Read the model definition and answer for the solid it produces. Units are mm, in the model's axes. A direction names the side the tool comes from. Coordinates: 2 decimals unless noted, no trailing zeros. Write each loop counter-clockwise with the first axis right and the second up, starting at its lowest first coordinate (ties: lowest second). Pieces come first, ordered by that corner, then holes. Notation, with made-up numbers: (62, 43.25) - (72, 43.25) arc R20 ccw to (72, 69.25) - close; hole circle Ø3 at (24, 59.25). An arc over 180 degrees is marked (long way). Return JSON: item names as keys, results as strings.
```python
from build123d import *

# Parameters (mm, degrees)
SKETCH_1_W      = 101
SKETCH_1_H      = 20
SKETCH_1_R      = 4
EXTRUDE_1_DEPTH = 3
EXTRUDE_2_DEPTH = 3
SKETCH_3_W      = 20
SKETCH_3_H      = 20
SKETCH_3_R      = 2
EXTRUDE_3_DEPTH = 3
SKETCH_4_W      = 95
SKETCH_4_H      = 20
EXTRUDE_4_DEPTH = 3
SKETCH_5_W      = 95
SKETCH_5_H      = 20
EXTRUDE_5_DEPTH = 3


with BuildPart() as part:
    # 草图1 → 凸台-拉伸1 (new body)
    with BuildSketch(Plane(origin=(0, 0, 0), x_dir=(1, 0, 0), z_dir=(0, 1, 0))):
        Rectangle(SKETCH_1_W, SKETCH_1_H)
        with Locations((-37.5, 0)):
            Circle(SKETCH_1_R, mode=Mode.SUBTRACT)
        with Locations((37.5, 0)):
            Circle(SKETCH_1_R, mode=Mode.SUBTRACT)
    extrude(amount=EXTRUDE_1_DEPTH)

    # 草图2 → 凸台-拉伸2 (add)
    with BuildSketch(Plane.ZY.offset(50.5)):
        Polygon((-10, 23), (-10, 3), (10, 3), (10, 23), (0, 23), align=None)
        with BuildLine():
            ThreePointArc((2, 13), (-1.414213562, 11.585786438), (0, 15))
            ThreePointArc((0, 15), (1.414213562, 14.414213562), (2, 13))
        make_face(mode=Mode.SUBTRACT)
    extrude(amount=-EXTRUDE_2_DEPTH)

    # 草图3 → 凸台-拉伸3 (add)
    with BuildSketch(Plane(origin=(50.5, 0, 0), x_dir=(0, 0, -1), z_dir=(1, 0, 0))):
        with Locations((0, 13)):
            Rectangle(SKETCH_3_W, SKETCH_3_H)
        with Locations((0, 13)):
            Circle(SKETCH_3_R, mode=Mode.SUBTRACT)
    extrude(amount=-EXTRUDE_3_DEPTH)

    # 草图4 → 凸台-拉伸4 (add)
    with BuildSketch(Plane.XY.offset(10)):
        with Locations((0, 13)):
            Rectangle(SKETCH_4_W, SKETCH_4_H)
    extrude(amount=-EXTRUDE_4_DEPTH)

    # 草图5 → 凸台-拉伸5 (add)
    with BuildSketch(Plane(origin=(0, 0, -10), x_dir=(-1, 0, 0), z_dir=(0, 0, -1))):
        with Locations((0, 13)):
            Rectangle(SKETCH_5_W, SKETCH_5_H)
    extrude(amount=-EXTRUDE_5_DEPTH)


solid = part.part
```
(1) A cutting plane is placed at C-C (z = 5.5). Determine the outline of the cut face in (x, y), and give its area (3 significant figures).
Answer:
{"outline": "(-50.5, 0) - (50.5, 0) - (50.5, 23) - (47.5, 23) - (47.5, 3) - (-47.5, 3) - (-47.5, 23) - (-50.5, 23) - close", "area": "423 mm²"}
(2) Determine the mould class of faces 1 (the face through (49, 15, 0)), 2 (the face through (-47.5, 15.4, -0.1)), 3 (the face through (-50.5, 12, 2)) for opening direction X: +X half, -X half, draft (parallel to the pull), parting line (faces both ways), or undercut.
Answer:
{"face 1": "draft", "face 2": "undercut", "face 3": "-X half"}
(3) A cutting plane is placed at D-D (x = -36). Determine the outline of the cut face in (y, z), and give its area (3 significant figures).
Answer:
{"outline": "(0, -10) - (23, -10) - (23, -7) - (3, -7) - (3, -3.71) - (0, -3.71) - close; (0, 3.71) - (3, 3.71) - (3, 7) - (23, 7) - (23, 10) - (0, 10) - close", "area": "158 mm²"}
(4) A flat-ended cylindrical pin translates along its axis: P1, Ø7, axis at x = 21.5, z = 1.5, coming from the +Y side. Find the tip coordinate at first contact, or state that the pin passes through.
Answer:
{"P1": "y = 3"}
(5) A cutting plane is placed at B-B (x = 37.5). Determine the outline of the cut face in (y, z), and give its area (3 significant figures).
Answer:
{"outline": "(0, -10) - (23, -10) - (23, -7) - (3, -7) - (3, -4) - (0, -4) - close; (0, 4) - (3, 4) - (3, 7) - (23, 7) - (23, 10) - (0, 10) - close", "area": "156 mm²"}
(6) A cutting plane is placed at A-A (y = 17.5). Determine the outline of the cut face in (x, z), and give its area (3 significant figures).
Answer:
{"outline": "(-50.5, -10) - (50.5, -10) - (50.5, 10) - (-50.5, 10) - close; hole (-47.5, -7) - (47.5, -7) - (47.5, 7) - (-47.5, 7) - close", "area": "690 mm²"}
(7) Which of the six approach directions +Z, -Z, +X, -X, +Y, -Y give full straight-line access (tool end or side, diameter ignored) to faces 4 (the face through (47.5, 15.4, 0.1)), 5 (the face through (-40.7, 1.5, 2.4))?
Answer:
{"face 4": "+Y", "face 5": "+Y, -Y"}
(8) Straight lines are drawn through the part: line 1 (Z direction, x = 3.5, y = 16.5); line 2 (X direction, y = 9.75, z = 2.5); line 3 (Y direction, x = -48.9, z = 0). For each, find the intervals that lie inside material, in ascending order. Write a range as from..to.
Answer:
{"line 1": "-10..-7, 7..10", "line 2": "-50.5..-47.5, 47.5..50.5", "line 3": "0..11, 15..23"}
